```python
from build123d import *

# Parameters (mm, degrees)
F0_R     = 11.25
F0_R_2   = 11.1
F1_DEPTH = 7
F2_R     = 2


with BuildPart() as f1:
    # F0 (on Top) → F1 (new body)
    with BuildSketch(Plane.XY):
        with BuildLine():
            ThreePointArc((4.282726, 12.041891), (-1.773401, 10.038879), (-7.829528, 12.041891))
            ThreePointArc((-7.829528, 12.041891), (-31.74895, -0.85611), (-6.51548, -10.944179))
            ThreePointArc((-6.51548, -10.944179), (-1.773401, -9.069235), (2.968677, -10.944179))
            ThreePointArc((2.968677, -10.944179), (28.202148, -0.85611), (4.282726, 12.041891))
        make_face()
        with Locations((-16.773401, 0)):
            Circle(F0_R, mode=Mode.SUBTRACT)
        with Locations((13.226599, 0)):
            Circle(F0_R_2, mode=Mode.SUBTRACT)
    extrude(amount=F1_DEPTH)

    # F2
    f2_edges = [f1.edges().sort_by_distance(p)[0] for p in [
        (-31.74895, -0.85611, 0),
        (28.202148, -0.85611, 7),
    ]]
    fillet(f2_edges, radius=F2_R)


solid = f1.part
```
Here's how the part is built. I have some questions about the finished solid (model axes, mm). Round coordinates to 2 decimals unless told otherwise and drop trailing zeros. Answer as CSV lines item,"result".
Item 1: Please list where these lines run through material, in increasing order: L1, parallel to X at y = 0.5, z = 2.75; L2, parallel to X at y = 9, z = 3.25; L3, parallel to Y at x = 15.5, z = 2.5. Write a range as [from, to].
From the geometry:
L1,"[-31.77, -28.01], [-5.53, 2.14], [24.32, 28.22]"
L2,"[-28.77, -23.52], [-10.02, 6.73], [19.72, 25.23]"
L3,"[-14.83, -10.86], [10.86, 14.83]"
Item 2: We'd pull the mould along Y, two halves only. Please class faces 1 (the flat face through (-2, 0, 7)), 2 (the cylindrical face through (-1.85, -9.07, 3.48)), 3 (the cylindrical face through (-25.7, -6.85, 3.45)): +Y half, -Y half, draft (parallel to the pull), parting line (faces both ways), or undercut.
From the geometry:
face 1,"draft"
face 2,"-Y half"
face 3,"undercut"
Item 3: For pin 1 (4 mm diameter, centred on y = -7, z = 6, fed in from -X); pin 2 (1.5 mm diameter, centred on x = -14.5, z = 5, fed in from +Y); pin 3 (4 mm diameter, centred on y = -7, z = 2, fed in from -X), each with a flat end and sliding along its axis, tell me the tip position at first contact or that it passes through.
From the geometry:
pin 1,"x = -30.85"
pin 2,"y = 14.92"
pin 3,"x = -30.92"
Item 4: Imagine slicing it at A-A on y = 0. Give the number of separate pieces and of enclosed holes in the cut face, and give its area (3 significant figures).
From the geometry:
separate pieces,"3"
enclosed holes,"0"
area,"104 mm2"
